Print and shaded views of the part. All mm, measured from the part's lowest x, y and z. Coordinates: 2 decimals unless noted, no trailing zeros. Order: outer loops, then holes, each group sorted by start corner. A loop starts at its lowest first (then second) coordinate and runs counter-clockwise, first axis right, second up.
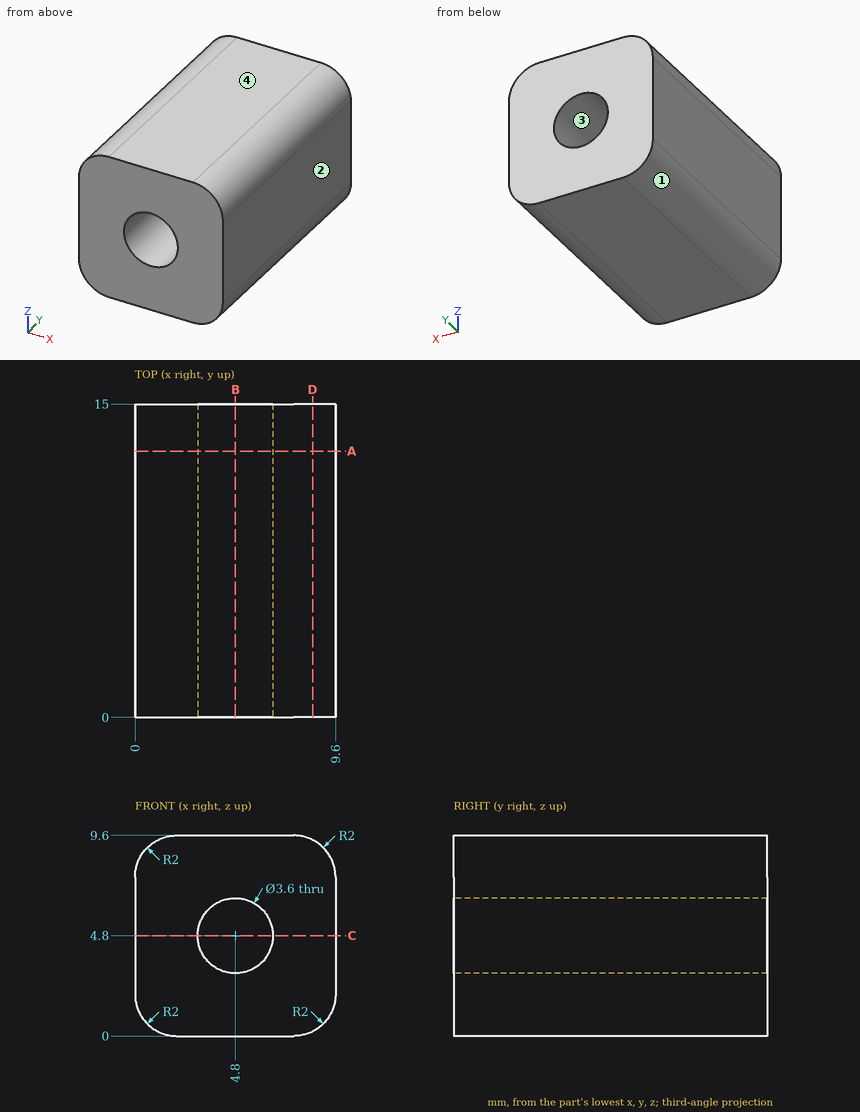
Q1. Cut at B-B, the plane x = 4.8. List the corners of the cut face in (y, z), plus the area to 3 significant figures.
Established:
outline: (0, 0) - (15, 0) - (15, 3) - (0, 3) - close; (0, 6.6) - (15, 6.6) - (15, 9.6) - (0, 9.6) - close
area: 90.0 mm2
Q2. Cut at C-C, the plane z = 4.8. List the corners of the cut face in (x, y).
Established:
outline: (0, 0) - (3, 0) - (3, 15) - (0, 15) - close; (6.6, 0) - (9.6, 0) - (9.6, 15) - (6.6, 15) - close
Q3. Probe line 1 (Z direction, x = 4.8, y = 6.75); line 2 (X direction, y = 5, z = 6); line 3 (Z direction, x = 4.25, y = 12.75). List the from-to ranges inside material, lowest first.
Established:
line 1: z = 0 to 3, 6.6 to 9.6
line 2: x = 0 to 3.46, 6.14 to 9.6
line 3: z = 0 to 3.09, 6.51 to 9.6
Q4. Cut at D-D, the plane x = 8.5. List the corners of the cut face in (y, z), plus the area to 3 significant figures.
Established:
outline: (0, 0.21) - (15, 0.21) - (15, 9.39) - (0, 9.39) - close
area: 138 mm2
Q5. Mould opens along Z. For the marked faces 1, 2, 3 and 4 say: pulls with the +Z half, pulls with the -Z half, needs draft (parallel to the pull), parting line crosses it, or undercut.
Established:
face 1: pulls with the -Z half
face 2: needs draft
face 3: undercut
face 4: pulls with the +Z half
Q6. Cut at A-A, the plane y = 12.75. List the corners of the cut face in (x, z).
Established:
outline: (0, 2) arc R2 ccw to (2, 0) - (7.6, 0) arc R2 ccw to (9.6, 2) - (9.6, 7.6) arc R2 ccw to (7.6, 9.6) - (2, 9.6) arc R2 ccw to (0, 7.6) - close; hole circle Ø3.6 at (4.8, 4.8)
Q7. Drop a flat-ended pin along its axis: P1, Ø2, axis at x = 4.8, z = 4.8, coming from the -Y side. Give the stop position or say it passes through.
Established:
P1: passes through
